```python
from build123d import *
from build123d.topology import SkipClean

# Parameters (mm, degrees)
SKETCH1_W           = 60
SKETCH1_H           = 41
BOSS_EXTRUDE1_DEPTH = 2
SKETCH2_R           = 9
CUT_EXTRUDE1_DEPTH  = 1
CUT_EXTRUDE2_DEPTH  = 1
SKETCH4_W           = 8
SKETCH4_H           = 8
CUT_EXTRUDE3_DEPTH  = 1
BOSS_EXTRUDE2_START = 5
BOSS_EXTRUDE2_DEPTH = 5
SKETCH6_R           = 1.6
CUT_EXTRUDE4_DEPTH  = 74.006848994
CHAMFER1_SIZE       = 1
CHAMFER2_SIZE       = 0.5
CHAMFER3_SIZE       = 1
FILLET1_R           = 2
BOSS_EXTRUDE3_DEPTH = 2.6
SKETCH8_W           = 2.5
SKETCH8_H           = 1
BOSS_EXTRUDE4_DEPTH = 5
FILLET2_R           = 2
BOSS_EXTRUDE5_START = 4
BOSS_EXTRUDE5_DEPTH = 4
SKETCH10_W          = 2.5
SKETCH10_H          = 7
BOSS_EXTRUDE6_DEPTH = 1.6


with BuildPart() as part:
    # Sketch1 → Boss-Extrude1 (new body)
    with BuildSketch(Plane.XY):
        with Locations((-30, 20.5)):
            Rectangle(SKETCH1_W, SKETCH1_H)
    extrude(amount=BOSS_EXTRUDE1_DEPTH)

    # Sketch2 → Cut-Extrude1 (cut)
    with BuildSketch(Plane.XY.offset(2)):
        with Locations((-49, 11)):
            Circle(SKETCH2_R)
        with Locations((-30, 11)):
            Circle(SKETCH2_R)
        with Locations((-11, 11)):
            Circle(SKETCH2_R)
        with Locations((-30, 30)):
            Circle(SKETCH2_R)
        with Locations((-11, 30)):
            Circle(SKETCH2_R)
        with Locations((-49, 30)):
            Circle(SKETCH2_R)
    extrude(amount=-CUT_EXTRUDE1_DEPTH, mode=Mode.SUBTRACT)

    # Sketch3 → Cut-Extrude2 (cut)
    with BuildSketch(Plane(origin=(0, 0, 0), x_dir=(-1, 0, 0), z_dir=(0, 0, -1))):
        with BuildLine():
            Line((54.5, 35.497915762), (54.5, 5.497915762))
            ThreePointArc((54.5, 5.497915762), (49, 1.895831523), (43.5, 5.497915762))
            Line((43.5, 5.497915762), (43.5, 35.497915762))
            ThreePointArc((43.5, 35.497915762), (49, 39.1), (54.5, 35.497915762))
        make_face()
        with BuildLine():
            Line((35.5, 35.497915762), (35.5, 5.497915762))
            ThreePointArc((35.5, 5.497915762), (30, 1.895831523), (24.5, 5.497915762))
            Line((24.5, 5.497915762), (24.5, 35.497915762))
            ThreePointArc((24.5, 35.497915762), (30, 39.1), (35.5, 35.497915762))
        make_face()
        with BuildLine():
            Line((16.5, 35.497915762), (16.5, 5.497915762))
            ThreePointArc((16.5, 5.497915762), (11, 1.895831523), (5.5, 5.497915762))
            Line((5.5, 5.497915762), (5.5, 35.497915762))
            ThreePointArc((5.5, 35.497915762), (11, 39.1), (16.5, 35.497915762))
        make_face()
    extrude(amount=-CUT_EXTRUDE2_DEPTH, mode=Mode.SUBTRACT)

    # Sketch4 → Cut-Extrude3 (cut)
    with BuildSketch(Plane(origin=(0, 0, 0), x_dir=(-1, 0, 0), z_dir=(0, 0, -1))):
        with Locations((39.5, 20.506096576)):
            Rectangle(SKETCH4_W, SKETCH4_H)
    extrude(amount=-CUT_EXTRUDE3_DEPTH, mode=Mode.SUBTRACT)

    # Sketch5 → Boss-Extrude2 (add)
    with SkipClean():  # the faces are left unmerged after this step: merging them gives an invalid solid
        with BuildSketch(Plane.XY.offset(2).offset(BOSS_EXTRUDE2_START)):
            with BuildLine():
                Line((-49, 20), (-49, 21))
                ThreePointArc((-49, 21), (-42.636038969, 23.636038969), (-40, 30))
                Line((-40, 30), (-39, 30))
                ThreePointArc((-39, 30), (-36.363961031, 23.636038969), (-30, 21))
                ThreePointArc((-30, 21), (-23.636038969, 23.636038969), (-21, 30))
                Line((-21, 30), (-20, 30))
                ThreePointArc((-20, 30), (-17.363961031, 23.636038969), (-11, 21))
                Line((-11, 21), (-11, 20))
                ThreePointArc((-11, 20), (-17.363961031, 17.363961031), (-20, 11))
                Line((-20, 11), (-21, 11))
                ThreePointArc((-21, 11), (-23.636038969, 17.363961031), (-30, 20))
                ThreePointArc((-30, 20), (-36.363961031, 17.363961031), (-39, 11))
                Line((-39, 11), (-40, 11))
                ThreePointArc((-40, 11), (-42.636038969, 17.363961031), (-49, 20))
            make_face()
            with BuildLine():
                Line((-2, 30), (0, 30))
                Line((0, 30), (0, 41))
                Line((0, 41), (-11, 41))
                Line((-11, 41), (-11, 39))
                ThreePointArc((-11, 39), (-4.636038969, 36.363961031), (-2, 30))
            make_face()
            with BuildLine():
                Line((-2, 11), (0, 11))
                Line((0, 11), (0, 0))
                Line((0, 0), (-11, 0))
                Line((-11, 0), (-11, 2))
                ThreePointArc((-11, 2), (-4.636038969, 4.636038969), (-2, 11))
            make_face()
            with BuildLine():
                Line((-49, 2), (-49, 0))
                Line((-49, 0), (-60, 0))
                Line((-60, 0), (-60, 11))
                Line((-60, 11), (-58, 11))
                ThreePointArc((-58, 11), (-55.363961031, 4.636038969), (-49, 2))
            make_face()
            with BuildLine():
                Line((-58, 30), (-60, 30))
                Line((-60, 30), (-60, 41))
                Line((-60, 41), (-49, 41))
                Line((-49, 41), (-49, 39))
                ThreePointArc((-49, 39), (-55.363961031, 36.363961031), (-58, 30))
            make_face()
        extrude(amount=-BOSS_EXTRUDE2_DEPTH)

    # Sketch6 → Cut-Extrude4 (cut, through all)
    with SkipClean():  # the faces are left unmerged after this step: merging them gives an invalid solid
        with BuildSketch(Plane.XY.offset(7)):
            with Locations((-39.5, 20.5)):
                Circle(SKETCH6_R)
            with Locations((-20.5, 20.5)):
                Circle(SKETCH6_R)
            with Locations((-2.75, 2.75)):
                Circle(SKETCH6_R)
            with Locations((-2.75, 38.25)):
                Circle(SKETCH6_R)
            with Locations((-57.25, 38.25)):
                Circle(SKETCH6_R)
            with Locations((-57.25, 2.75)):
                Circle(SKETCH6_R)
        extrude(amount=-CUT_EXTRUDE4_DEPTH, mode=Mode.SUBTRACT)

    # Chamfer1
    chamfer1_edges = [part.edges().sort_by_distance(p)[0] for p in [
        (-22.1, 20.5, 0),
        (-41.1, 20.5, 1),
    ]]
    chamfer(chamfer1_edges, length=CHAMFER1_SIZE)

    # Chamfer2
    # the kernel refuses this chamfer: 0.5 mm, written as the material it takes off along each edge
    with BuildSketch(Plane(origin=(-39, 30, 8.324152825), x_dir=(-1, 0, 0), z_dir=(0, 0, -1)), Plane(origin=(-49, 21, 8.324152825), x_dir=(0, -1, 0), z_dir=(0, 0, -1)), Plane(origin=(-40, 11, 8.324152825), x_dir=(1, 0, 0), z_dir=(0, 0, -1)), Plane(origin=(-21, 11, 8.324152825), x_dir=(1, 0, 0), z_dir=(0, 0, -1)), Plane(origin=(-11, 20, 8.324152825), x_dir=(0, 1, 0), z_dir=(0, 0, -1)), Plane(origin=(-20, 30, 8.324152825), x_dir=(-1, 0, 0), z_dir=(0, 0, -1))) as chamfer2_piece_1:
        with BuildLine():
            Line((CHAMFER2_SIZE, 0), (-0.014731413, -0.514731413))
            ThreePointArc((-0.014731413, -0.514731413), (-0.003894786, -0.264747015), (0, 0))
            Line((0, 0), (CHAMFER2_SIZE, 0))
        make_face()
    extrude(amount=6.324152825, mode=Mode.SUBTRACT)
    with BuildSketch(Plane(origin=(-40, 30, 8.324152825), x_dir=(1, 0, 0), z_dir=(0, 0, -1)), Plane(origin=(-49, 20, 8.324152825), x_dir=(0, 1, 0), z_dir=(0, 0, -1)), Plane(origin=(-39, 11, 8.324152825), x_dir=(-1, 0, 0), z_dir=(0, 0, -1)), Plane(origin=(-20, 11, 8.324152825), x_dir=(-1, 0, 0), z_dir=(0, 0, -1)), Plane(origin=(-11, 21, 8.324152825), x_dir=(0, -1, 0), z_dir=(0, 0, -1)), Plane(origin=(-21, 30, 8.324152825), x_dir=(1, 0, 0), z_dir=(0, 0, -1))) as chamfer2_piece_2:
        with BuildLine():
            Line((CHAMFER2_SIZE, 0), (-0.014731413, 0.514731413))
            ThreePointArc((-0.014731413, 0.514731413), (-0.003894786, 0.264747015), (0, 0))
            Line((0, 0), (CHAMFER2_SIZE, 0))
        make_face()
    extrude(amount=6.324152825, mode=Mode.SUBTRACT)

    # Chamfer3
    # the kernel refuses this chamfer: 1 mm, written as the material it takes off along each edge
    with BuildSketch(Plane(origin=(-49, 39, 9.73772815), x_dir=(0, 1, 0), z_dir=(0, 0, -1)), Plane(origin=(-2, 30, 9.73772815), x_dir=(1, 0, 0), z_dir=(0, 0, -1)), Plane(origin=(-11, 2, 9.73772815), x_dir=(0, -1, 0), z_dir=(0, 0, -1)), Plane(origin=(-58, 11, 9.73772815), x_dir=(-1, 0, 0), z_dir=(0, 0, -1))) as chamfer3_piece_1:
        with BuildLine():
            Line((CHAMFER3_SIZE, 0), (-0.062996063, -1.062996063))
            ThreePointArc((-0.062996063, -1.062996063), (-0.016662827, -0.547405922), (0, 0))
            Line((0, 0), (CHAMFER3_SIZE, 0))
        make_face()
    extrude(amount=7.73772815, mode=Mode.SUBTRACT)
    with BuildSketch(Plane(origin=(-49, 41, 9.571682988), x_dir=(-1, 0, 0), z_dir=(0, 0, -1)), Plane(origin=(0, 30, 9.571682988), x_dir=(0, 1, 0), z_dir=(0, 0, -1)), Plane(origin=(-11, 0, 9.571682988), x_dir=(1, 0, 0), z_dir=(0, 0, -1)), Plane(origin=(-60, 11, 9.571682988), x_dir=(0, -1, 0), z_dir=(0, 0, -1))) as chamfer3_piece_2:
        Polygon((CHAMFER3_SIZE, 0), (0, -CHAMFER3_SIZE), (0, 0), align=None)
    extrude(amount=7.571682988, mode=Mode.SUBTRACT)
    with BuildSketch(Plane(origin=(-11, 39, 9.73772815), x_dir=(0, 1, 0), z_dir=(0, 0, -1)), Plane(origin=(-2, 11, 9.73772815), x_dir=(1, 0, 0), z_dir=(0, 0, -1)), Plane(origin=(-49, 2, 9.73772815), x_dir=(0, -1, 0), z_dir=(0, 0, -1)), Plane(origin=(-58, 30, 9.73772815), x_dir=(-1, 0, 0), z_dir=(0, 0, -1))) as chamfer3_piece_3:
        with BuildLine():
            Line((CHAMFER3_SIZE, 0), (-0.062996063, 1.062996063))
            ThreePointArc((-0.062996063, 1.062996063), (-0.016662827, 0.547405922), (0, 0))
            Line((0, 0), (CHAMFER3_SIZE, 0))
        make_face()
    extrude(amount=7.73772815, mode=Mode.SUBTRACT)
    with BuildSketch(Plane(origin=(-11, 41, 9.571682988), x_dir=(1, 0, 0), z_dir=(0, 0, -1)), Plane(origin=(0, 11, 9.571682988), x_dir=(0, -1, 0), z_dir=(0, 0, -1)), Plane(origin=(-49, 0, 9.571682988), x_dir=(-1, 0, 0), z_dir=(0, 0, -1)), Plane(origin=(-60, 30, 9.571682988), x_dir=(0, 1, 0), z_dir=(0, 0, -1))) as chamfer3_piece_4:
        Polygon((CHAMFER3_SIZE, 0), (0, CHAMFER3_SIZE), (0, 0), align=None)
    extrude(amount=7.571682988, mode=Mode.SUBTRACT)

    # Fillet1
    fillet1_edges = [part.edges().sort_by_distance(p)[0] for p in [
        (0, 0, 3.5),
        (-60, 0, 3.5),
        (-60, 41, 3.5),
        (0, 41, 3.5),
    ]]
    fillet(fillet1_edges, radius=FILLET1_R)

    # Sketch7 → Boss-Extrude3 (add)
    with BuildSketch(Plane(origin=(0, 0, 0), x_dir=(-1, 0, 0), z_dir=(0, -1, 0))):
        Polygon((5.5, -7), (7.5, -7), (7.5, -2), (10, -2), (10, 0), (7.5, 0), (5.5, 0), align=None)
        Polygon((50, 0), (52.5, 0), (54.5, 0), (54.5, -7), (52.5, -7), (52.5, -2), (50, -2), align=None)
    extrude(amount=BOSS_EXTRUDE3_DEPTH)

    # Sketch8 → Boss-Extrude4 (add)
    with BuildSketch(Plane.XY.offset(2)):
        with Locations((-8.75, -2.1)):
            Rectangle(SKETCH8_W, SKETCH8_H)
        with Locations((-51.25, -2.1)):
            Rectangle(SKETCH8_W, SKETCH8_H)
    extrude(amount=BOSS_EXTRUDE4_DEPTH)

    # Fillet2
    fillet2_edges = [part.edges().sort_by_distance(p)[0] for p in [
        (-5.5, -2.6, 3.5),
        (-54.5, -2.6, 3.5),
    ]]
    fillet(fillet2_edges, radius=FILLET2_R)

    # Sketch9 → Boss-Extrude5 (add)
    with BuildSketch(Plane.XY.offset(7).offset(BOSS_EXTRUDE5_START)):
        with BuildLine():
            Line((-5.5, 0), (-7.5, 0))
            Line((-7.5, 0), (-7.5, -1.6))
            Line((-7.5, -1.6), (-10, -1.6))
            Line((-10, -1.6), (-10, -2.6))
            Line((-10, -2.6), (-7.5, -2.6))
            ThreePointArc((-7.5, -2.6), (-6.085786438, -2.014213562), (-5.5, -0.6))
            Line((-5.5, -0.6), (-5.5, 0))
        make_face()
        with BuildLine():
            ThreePointArc((-52.5, -2.6), (-53.914213562, -2.014213562), (-54.5, -0.6))
            Line((-54.5, -0.6), (-54.5, 0))
            Line((-54.5, 0), (-52.5, 0))
            Line((-52.5, 0), (-52.5, -1.6))
            Line((-52.5, -1.6), (-50, -1.6))
            Line((-50, -1.6), (-50, -2.6))
            Line((-50, -2.6), (-52.5, -2.6))
        make_face()
    extrude(amount=-BOSS_EXTRUDE5_DEPTH)

    # Sketch10 → Boss-Extrude6 (add)
    with BuildSketch(Plane(origin=(0, -1.6, 0), x_dir=(1, 0, 0), z_dir=(0, 1, 0))):
        with Locations((-8.75, -5.5)):
            Rectangle(SKETCH10_W, SKETCH10_H)
        with Locations((-51.25, -5.5)):
            Rectangle(SKETCH10_W, SKETCH10_H)
    extrude(amount=BOSS_EXTRUDE6_DEPTH)


solid = part.part
```
Could you check a few things on this model? Use its own coordinates, in mm. A direction names the side the tool comes from. Coordinates: 2 decimals unless noted, no trailing zeros. Order: outer loops, then holes, each group sorted by start corner. A loop starts at its lowest first (then second) coordinate and runs counter-clockwise, first axis right, second up. Notation, with made-up numbers: M 37,39.5 L 55,39.5 A22 ccw 55,55.5 Z; hole C 88,47.25 d10. An arc over 180 degrees is marked long. Use a Markdown table: item, result. Add a question column.
Q1. I'm going to push flat-ended pins straight in: pin 1 (1.8 mm diameter, centred on y = -1, z = 10.5, fed in from +X); pin 2 (9 mm diameter, centred on x = -31.5, y = 33.5, fed in from +Z); pin 3 (9 mm diameter, centred on x = -4.5, y = 16, fed in from +Z); pin 4 (1 mm diameter, centred on x = -31, y = 23.5, fed in from -Z). Where does each tip first touch, or does it pass through?
Q2. I want a section at B-B on z = 6.25. Give the number of separate pieces and of enclosed holes in the cut face, then the cut area to 3 significant figures.
Q3. We'd pull the mould along X, two halves only. Please class faces 1 (the flat face through (-37, 10, 1)), 2 (the cylindrical face through (-53.9, -2.03, 5.58)), 3 (the flat face through (-29.9, 20.5, 7)), 4 (the cylindrical face through (-55.77, 37.64, 3.55)): pulls with the +X half, pulls with the -X half, needs draft (parallel to the pull), parting line crosses it, or undercut.
Q4. I want a section at C-C on y = 34.5. List the corners of the cut face in (x, z) for me.
Q5. I want a section at A-A on z = 9.75. List the corners of the cut face in (x, y) for me, then the cut area to 3 significant figures.
Q6. Which directions (+Z, -Z, +X, -X, +Y, -Y) give clear straight access to the entire face, cutting with the end or side of a thin tool? Please do faces 5 (the flat face through (-18, 30, 1)), 6 (the flat face through (-51, -1, 9)), 7 (the flat face through (-30, 0, 1)).
Q7. I want a section at D-D on y = 7.5. List the corners of the cut face in (x, z) for me.
Q8. If I drill on L1, parallel to Y at x = -11, z = 1.6; L2, parallel to X at y = 30, z = 1.25; L3, parallel to Y at x = -3, z = 4.5, over which ranges is the centre line in solid material (lowest first)?
Checked values:
| question | item | result |
|---|---|---|
| 1 | pin 1 | x = -5.5 |
| 1 | pin 2 | z = 1 |
| 1 | pin 3 | z = 2 |
| 1 | pin 4 | through |
| 2 | separate pieces | 5 |
| 2 | enclosed holes | 6 |
| 2 | area | 403 mm² |
| 3 | face 1 | undercut |
| 3 | face 2 | pulls with the -X half |
| 3 | face 3 | needs draft |
| 3 | face 4 | undercut |
| 4 | outline | M -60,0 L -54.5,0 L -54.5,1 L -56.79,1 L -56.79,7 L -60,7 Z; M -43.5,0 L -35.5,0 L -35.5,1 L -37.79,1 L -37.79,2 L -41.21,2 L -41.21,1 L -43.5,1 Z; M -24.5,0 L -16.5,0 L -16.5,1 L -18.79,1 L -18.79,2 L -22.21,2 L -22.21,1 L -24.5,1 Z; M -5.5,0 L 0,0 L 0,7 L -3.21,7 L -3.21,1 L -5.5,1 Z |
| 5 | outline | M -54.5,-0.6 A2 ccw -52.5,-2.6 L -50,-2.6 L -50,-1.6 L -52.5,-1.6 L -52.5,0 L -54.5,0 Z; M -10,-2.6 L -7.5,-2.6 A2 ccw -5.5,-0.6 L -5.5,0 L -7.5,0 L -7.5,-1.6 L -10,-1.6 Z |
| 5 | area | 13.7 mm² |
| 6 | face 5 | +Z |
| 6 | face 6 | +Z, +Y |
| 6 | face 7 | +Z, -Z, -Y |
| 7 | outline | M -60,0 L -54.5,0 L -54.5,1 L -57.29,1 L -57.29,7 L -60,7 Z; M -43.5,0 L -35.5,0 L -35.5,1 L -38.29,1 L -38.29,2 L -40.71,2 L -40.71,1 L -43.5,1 Z; M -24.5,0 L -16.5,0 L -16.5,1 L -19.29,1 L -19.29,2 L -21.71,2 L -21.71,1 L -24.5,1 Z; M -5.5,0 L 0,0 L 0,7 L -2.71,7 L -2.71,1 L -5.5,1 Z |
| 8 | L1 | 0 to 2, 20 to 21, 39 to 41 |
| 8 | L2 | -60 to -58, -40 to -39, -21 to -20, -2 to 0 |
| 8 | L3 | 0 to 1.17, 4.33 to 6.88, 34.12 to 36.67, 39.83 to 41 |
